from build123d import *

# Parameters (mm, degrees)
SKETCH1_R           = 8.5
BOSS_EXTRUDE1_DEPTH = 1.9
BOSS_EXTRUDE2_DEPTH = 1.9
CIRPATTERN2_COUNT   = 12
FILLET5_R           = 6
FILLET6_R           = 6
BOSS_EXTRUDE5_DEPTH = 1.9
SKETCH15_R          = 5
BOSS_EXTRUDE6_DEPTH = 1.9
SKETCH14_R          = 1.5
CUT_EXTRUDE7_DEPTH  = 24.297043988
CUT_EXTRUDE8_DEPTH  = 24.297043988
SKETCH17_R          = 1.5
CUT_EXTRUDE9_DEPTH  = 24.297043988
FILLET7_R           = 2.5


# Some blends are built 0.0001 mm under size
with BuildPart() as part:
    # Sketch1 → Boss-Extrude1 (new body)
    with BuildSketch(Plane.XY):
        with Locations(Location((0, 0, 0), (0, 0, 180))):
            Circle(SKETCH1_R)
    extrude(amount=BOSS_EXTRUDE1_DEPTH)

    # Sketch3 → Boss-Extrude2 (add)
    with BuildSketch(Plane.XY.offset(1.9)):
        Polygon((-1.305261922, 9.914448614), (-1.509060022, 7), (1.509060022, 7), (1.305261922, 9.914448614), (0.678518537, 11), (-0.678518537, 11), align=None)
    boss_extrude2 = extrude(amount=-BOSS_EXTRUDE2_DEPTH)

    # CirPattern2: Boss-Extrude2 ×12 about axis
    cirpattern2_axis = Axis((0, 0, 0), (0, 0, 1))
    for i in range(1, CIRPATTERN2_COUNT):
        add(boss_extrude2.rotate(cirpattern2_axis, i * 360 / CIRPATTERN2_COUNT))

    # Fillet5
    # the kernel refuses this fillet: 6 mm, written as the material it takes off along each edge
    with BuildSketch(Plane(origin=(9.238795325, 3.826834324, 5.354382408), x_dir=(0.49999999999981276, 0.8660254037845467, 0), z_dir=(0, 0, -1)), Plane(origin=(1.305261922, 9.914448614, 5.354382408), x_dir=(-0.5000000000001841, 0.8660254037843323, 0), z_dir=(0, 0, -1)), Plane(origin=(-7.933533403, 6.08761429, 5.354382408), x_dir=(-1, 0, 0), z_dir=(0, 0, -1)), Plane(origin=(-9.914448614, 1.305261922, 5.354382408), x_dir=(-0.8660254037843321, -0.5000000000001844, 0), z_dir=(0, 0, -1)), Plane(origin=(-9.238795325, -3.826834324, 5.354382408), x_dir=(-0.49999999999981826, -0.8660254037845436, 0), z_dir=(0, 0, -1)), Plane(origin=(-6.08761429, -7.933533403, 5.354382408), x_dir=(0, -1, 0), z_dir=(0, 0, -1)), Plane(origin=(3.826834324, -9.238795325, 5.354382408), x_dir=(0.8660254037845474, -0.49999999999981154, 0), z_dir=(0, 0, -1)), Plane(origin=(7.933533403, -6.08761429, 5.354382408), x_dir=(1, 0, 0), z_dir=(0, 0, -1)), Plane(origin=(9.914448614, -1.305261922, 5.354382408), x_dir=(0.866025403784333, 0.500000000000183, 0), z_dir=(0, 0, -1))) as fillet5_piece_1:
        with BuildLine():
            CenterArc((1.388315544, -5.998484909), FILLET5_R, 91.287628333, 24.712371667)
            Line((-1.241911337, -0.605720631), (-1.294515874, -0.497865346))
            Line((-1.294515874, -0.497865346), (-0.052604538, 0.107855286))
            Line((-0.052604538, 0.107855286), (0, 0.12))
            ThreePointArc((0, 0.12), (0.626743385, 0.12), (1.250790195, 0.119969698))
            Line((1.250790195, 0.119969698), (1.25348677, 0))
        make_face()
    extrude(amount=8.808764816, mode=Mode.SUBTRACT)
    with BuildSketch(Plane(origin=(6.08761429, 7.933533403, 5.354382408), x_dir=(-0.4383711467890806, -0.8987940462991654, 0), z_dir=(0, 0, -1)), Plane(origin=(-3.826834324, 9.238795325, 5.354382408), x_dir=(0.5591929034707432, -0.8290375725550441, 0), z_dir=(0, 0, -1)), Plane(origin=(-1.305261922, -9.914448614, 5.354382408), x_dir=(-0.06975647374412203, 0.9975640502598244, 0), z_dir=(0, 0, -1))) as fillet5_piece_2:
        with BuildLine():
            CenterArc((1.381752963, 6), FILLET5_R, 245.287628333, 24.712371667)
            Line((-1.126626446, 0.549492433), (-1.176794034, 0.440482282))
            ThreePointArc((-1.176794034, 0.440482282), (-0.615917761, 0.166890931), (-0.052604538, -0.107855286))
            Line((-0.052604538, -0.107855286), (0, -0.12))
            Line((0, -0.12), (1.381752963, -0.12))
            Line((1.381752963, -0.12), (1.381752963, 0))
        make_face()
    extrude(amount=8.808764816, mode=Mode.SUBTRACT)

    # Fillet6
    # the kernel refuses this fillet: 6 mm, written as the material it takes off along each edge
    with BuildSketch(Plane(origin=(7.933533403, 6.08761429, 5.354382408), x_dir=(-0.8987940462991681, -0.4383711467890751, 0), z_dir=(0, 0, -1)), Plane(origin=(3.826834324, 9.238795325, 5.354382408), x_dir=(-0.5591929034707512, -0.8290375725550386, 0), z_dir=(0, 0, -1)), Plane(origin=(-1.305261922, 9.914448614, 5.354382408), x_dir=(-0.06975647374412959, -0.9975640502598239, 0), z_dir=(0, 0, -1)), Plane(origin=(-6.08761429, 7.933533403, 5.354382408), x_dir=(0.43837114678907496, -0.8987940462991681, 0), z_dir=(0, 0, -1)), Plane(origin=(-9.238795325, 3.826834324, 5.354382408), x_dir=(0.8290375725550395, -0.5591929034707501, 0), z_dir=(0, 0, -1)), Plane(origin=(-9.914448614, -1.305261922, 5.354382408), x_dir=(0.9975640502598241, -0.0697564737441288, 0), z_dir=(0, 0, -1)), Plane(origin=(-7.933533403, -6.08761429, 5.354382408), x_dir=(0.8987940462991686, 0.4383711467890744, 0), z_dir=(0, 0, -1)), Plane(origin=(-3.826834324, -9.238795325, 5.354382408), x_dir=(0.5591929034707488, 0.8290375725550403, 0), z_dir=(0, 0, -1)), Plane(origin=(1.305261922, -9.914448614, 5.354382408), x_dir=(0.06975647374412966, 0.9975640502598239, 0), z_dir=(0, 0, -1)), Plane(origin=(6.08761429, -7.933533403, 5.354382408), x_dir=(-0.4383711467890749, 0.8987940462991683, 0), z_dir=(0, 0, -1)), Plane(origin=(9.238795325, -3.826834324, 5.354382408), x_dir=(-0.8290375725550393, 0.5591929034707505, 0), z_dir=(0, 0, -1)), Plane(origin=(9.914448614, 1.305261922, 5.354382408), x_dir=(-0.9975640502598239, 0.06975647374412894, 0), z_dir=(0, 0, -1))) as fillet6_piece_1:
        with BuildLine():
            CenterArc((1.381752963, -6), FILLET6_R, 90, 24.712371667)
            Line((-1.126626446, -0.549492433), (-1.176794034, -0.440482282))
            ThreePointArc((-1.176794034, -0.440482282), (-0.615917761, -0.166890931), (-0.052604538, 0.107855286))
            Line((-0.052604538, 0.107855286), (0, 0.12))
            Line((0, 0.12), (1.381752963, 0.12))
            Line((1.381752963, 0.12), (1.381752963, 0))
        make_face()
    extrude(amount=8.808764816, mode=Mode.SUBTRACT)

    # Sketch12 → Boss-Extrude5 (add)
    with BuildSketch(Plane(origin=(0, 0, 0), x_dir=(-1, 0, 0), z_dir=(0, 0, -1))):
        Polygon((1.535905814, 15.391336798), (-5.261824062, -9.978136476), (-0.43219493, -11.272231702), (7.72060499, 19.154431826), (2.890975859, 20.448527052), align=None)
    extrude(amount=-BOSS_EXTRUDE5_DEPTH)

    # Sketch15 → Boss-Extrude6 (add)
    with BuildSketch(Plane(origin=(0, 0, 0), x_dir=(-1, 0, 0), z_dir=(0, 0, -1))):
        Circle(SKETCH15_R)
    extrude(amount=-BOSS_EXTRUDE6_DEPTH)

    # Sketch14 → Cut-Extrude7 (cut, through all)
    with BuildSketch(Plane(origin=(0, 0, 0), x_dir=(-1, 0, 0), z_dir=(0, 0, -1))):
        Circle(SKETCH14_R)
    extrude(amount=-CUT_EXTRUDE7_DEPTH, mode=Mode.SUBTRACT)

    # Sketch16 → Cut-Extrude8 (cut, through all)
    with BuildSketch(Plane.XY.offset(1.9)):
        Polygon((-5.659024027, 11.460506927), (0.43219493, -11.272231702), (-8.69145043, -13.716905108), (-14.782669387, 9.015833521), align=None)
    extrude(amount=-CUT_EXTRUDE8_DEPTH, mode=Mode.SUBTRACT)

    # Sketch17 → Cut-Extrude9 (cut, through all)
    with BuildSketch(Plane.XY.offset(1.9)):
        with Locations((-4.658742812, 17.386664873)):
            Circle(SKETCH17_R)
    extrude(amount=-CUT_EXTRUDE9_DEPTH, mode=Mode.SUBTRACT)

    # Fillet7
    fillet7_edges = [part.edges().sort_by_distance(p)[0] for p in [
        (-7.72060499, 19.154431826, 0.95),
        (-2.890975859, 20.448527052, 0.95),
        (0.43219493, -11.272231702, 0.95),
    ]]
    fillet(fillet7_edges, radius=FILLET7_R - 0.0001)  # a hair under: the kernel refuses the full size


solid = part.part
Source: CAD feature listing. Evaluate the final solid. Frame: model axes, mm. A direction names the side the tool comes from. Coordinates: 2 decimals unless noted, no trailing zeros. Order: outer loops, then holes, each group sorted by start corner. A loop starts at its lowest first (then second) coordinate and runs counter-clockwise, first axis right, second up.
Item 1: First-contact query: P1, Ø0.5, axis at x = 0.5, z = 1, coming from the +Y side; P2, Ø5, axis at x = 1.5, y = 16, coming from the +Z side. Flat tips, straight axial feed; report the tip coordinate or a pass-through.
Output values:
P1: stops at y = 11
P2: passes through
Item 2: Cut plane C-C (z = 0.6). Count the separate pieces of the cut face and the enclosed holes in it, plus the area to 3 significant figures.
Output values:
separate pieces: 1
enclosed holes: 2
area: 240 mm2
Item 3: Material intervals for line 1 (Y direction, x = 9, z = 0.8); line 2 (X direction, y = 9.5, z = 1.3); line 3 (X direction, y = 17.5, z = 1.7), sorted ascending.
Output values:
line 1: y = -6.08 to -3.81, -1.35 to 1.35, 3.81 to 6.08
line 2: x = -5.13 to 1.25, 4.38 to 5.55
line 3: x = -7.16 to -6.15, -3.16 to -2.1
Item 4: Cut plane D-D (x = 3.5). Return loops of the section in (y, z), plus the area to 3 significant figures.
Output values:
outline: (-10.45, 0) - (8.67, 0) - (8.67, 1.9) - (-10.45, 1.9) - close
area: 36.3 mm2
Item 5: Set-up query: faces 1 (the face through (3.874, 9.067, 0.963)), 2 (the face through (9.067, -3.874, 0.963)), 3 (the face through (7.924, -5.924, 0.963)), 4 (the face through (6, -6.02, 0.94)), 5 (the face through (2, 1, 0)). Return all of +Z, -Z, +X, -X, +Y, -Y with unobstructed straight access to the full face (end or side cutting, diameter ignored); none if empty.
Output values:
face 1: +Z, -Z, +Y
face 2: +Z, -Z, +X
face 3: +Z, -Z, -Y
face 4: +Z, -Z
face 5: -Z, +X, -X, +Y, -Y
Item 6: Pull-direction query (X, two-part tool) for faces 6 (the face through (-3.967, 16.056, 0.963)), 7 (the face through (8.207, -2.211, 0.937)), 8 (the face through (-6.81, 18.66, 0.96)), 9 (the face through (2, 1, 1.9)); classes: pulls with the +X half, pulls with the -X half, needs draft (parallel to the pull), parting line crosses it, or undercut.
Output values:
face 6: undercut
face 7: pulls with the +X half
face 8: pulls with the -X half
face 9: needs draft
Item 7: Cut plane B-B (y = 0). Return loops of the section in (x, z), plus the area to 3 significant figures.
Output values:
outline: (-2.59, 0) - (-1.5, 0) - (-1.5, 1.9) - (-2.59, 1.9) - close; (1.5, 0) - (11, 0) - (11, 1.9) - (1.5, 1.9) - close
area: 20.1 mm2
Item 8: Cut plane A-A (x = -4.5). Return loops of the section in (y, z).
Output values:
outline: (7.13, 0) - (15.9, 0) - (15.9, 1.9) - (7.13, 1.9) - close; (18.88, 0) - (19.88, 0) - (19.88, 1.9) - (18.88, 1.9) - close
